from build123d import *

# Parameters (mm, degrees)
EXTRUDE_1_DEPTH     = 10
FILLET_1_R          = 20
SKETCH_2_R          = 18.75
CUT_EXTRUDE_1_DEPTH = 81.195074662
SKETCH_5_R          = 1.65
CUT_EXTRUDE_4_DEPTH = 81.195074662
SKETCH_6_R          = 1.65
CUT_EXTRUDE_5_DEPTH = 81.195074662
SKETCH_7_R          = 18.75
SKETCH_7_R_2        = 17.75
EXTRUDE_2_DEPTH     = 3
CUT_EXTRUDE_6_DEPTH = 10
FILLET_5_R          = 5
FILLET_6_R          = 3


with BuildPart() as part:
    # ｽｹｯﾁ1 → ﾎﾞｽ - 押し出し1 (new body)
    with BuildSketch(Plane.XY):
        with BuildLine():
            Line((57.5, -15), (57.5, 15))
            Line((57.5, 15), (48.35142739, 38.928092678))
            ThreePointArc((48.35142739, 38.928092678), (39.173878846, 50.59371648), (25, 55))
            Line((25, 55), (-25, 55))
            ThreePointArc((-25, 55), (-39.173878846, 50.59371648), (-48.35142739, 38.928092678))
            Line((-48.35142739, 38.928092678), (-57.5, 15))
            Line((-57.5, 15), (-57.5, -15))
            Line((-57.5, -15), (57.5, -15))
        make_face()
    extrude(amount=EXTRUDE_1_DEPTH)

    # ﾌｨﾚｯﾄ1
    fillet_1_edges = [part.edges().sort_by_distance(p)[0] for p in [
        (57.5, 15, 5),
        (-57.5, 15, 5),
    ]]
    fillet(fillet_1_edges, radius=FILLET_1_R)

    # ｽｹｯﾁ2 → ｶｯﾄ - 押し出し1 (cut, through all)
    with BuildSketch(Plane.XY.offset(10)):
        with Locations((25, 30)):
            Circle(SKETCH_2_R)
        with Locations(Location((-25, 30, 0), (0, 0, 180))):
            Circle(SKETCH_2_R)
    extrude(amount=-CUT_EXTRUDE_1_DEPTH, mode=Mode.SUBTRACT)

    # ｽｹｯﾁ5 → ｶｯﾄ - 押し出し4 (cut, through all)
    with BuildSketch(Plane(origin=(0, 0, 0), x_dir=(-1, 0, 0), z_dir=(0, 0, -1))):
        with Locations((-25, 51.75)):
            Circle(SKETCH_5_R)
        with Locations((-9.620427509, 45.379572491)):
            Circle(SKETCH_5_R)
        with Locations((-3.25, 30)):
            Circle(SKETCH_5_R)
        with Locations((-9.620427509, 14.620427509)):
            Circle(SKETCH_5_R)
        with Locations((-25, 8.25)):
            Circle(SKETCH_5_R)
        with Locations((-40.379572491, 14.620427509)):
            Circle(SKETCH_5_R)
        with Locations((-46.75, 30)):
            Circle(SKETCH_5_R)
        with Locations((-40.379572491, 45.379572491)):
            Circle(SKETCH_5_R)
        with Locations(Location((40.379572491, 45.379572491, 0), (0, 0, 180))):
            Circle(SKETCH_5_R)
        with Locations(Location((46.75, 30, 0), (0, 0, 180))):
            Circle(SKETCH_5_R)
        with Locations(Location((40.379572491, 14.620427509, 0), (0, 0, 180))):
            Circle(SKETCH_5_R)
        with Locations(Location((25, 8.25, 0), (0, 0, 180))):
            Circle(SKETCH_5_R)
        with Locations(Location((9.620427509, 14.620427509, 0), (0, 0, 180))):
            Circle(SKETCH_5_R)
        with Locations(Location((3.25, 30, 0), (0, 0, 180))):
            Circle(SKETCH_5_R)
        with Locations(Location((9.620427509, 45.379572491, 0), (0, 0, 180))):
            Circle(SKETCH_5_R)
        with Locations(Location((25, 51.75, 0), (0, 0, 180))):
            Circle(SKETCH_5_R)
    extrude(amount=-CUT_EXTRUDE_4_DEPTH, mode=Mode.SUBTRACT)

    # ｽｹｯﾁ6 → ｶｯﾄ - 押し出し5 (cut, through all)
    with BuildSketch(Plane(origin=(0, 0, 0), x_dir=(-1, 0, 0), z_dir=(0, 0, -1))):
        with Locations((-52.5, -5)):
            Circle(SKETCH_6_R)
        with Locations(Location((52.5, -5, 0), (0, 0, 180))):
            Circle(SKETCH_6_R)
        with Locations((0, -5)):
            Circle(SKETCH_6_R)
    extrude(amount=-CUT_EXTRUDE_5_DEPTH, mode=Mode.SUBTRACT)

    # ｽｹｯﾁ7 → ﾎﾞｽ - 押し出し2 (add)
    # profile 1 of 2: a face of its own
    with BuildSketch(Plane.XY.offset(10)):
        with Locations((-25, 30)):
            Circle(SKETCH_7_R)
        with Locations((-25, 30)):
            Circle(SKETCH_7_R_2, mode=Mode.SUBTRACT)
    # profile 2 of 2: a face of its own
    with BuildSketch(Plane.XY.offset(10)):
        with Locations((25, 30)):
            Circle(SKETCH_7_R)
        with Locations((25, 30)):
            Circle(SKETCH_7_R_2, mode=Mode.SUBTRACT)
    extrude(amount=-EXTRUDE_2_DEPTH)

    # ｽｹｯﾁ8 → ｶｯﾄ - 押し出し6 (cut)
    with BuildSketch(Plane(origin=(0, 0, 0), x_dir=(-1, 0, 0), z_dir=(0, 0, -1))):
        with BuildLine():
            Line((-42.5, -9), (-7.5, -9))
            Line((-7.5, -9), (-7.5, 8.786796564))
            ThreePointArc((-7.5, 8.786796564), (-25, 2.5), (-42.5, 8.786796564))
            Line((-42.5, 8.786796564), (-42.5, -9))
        make_face()
        with BuildLine():
            Line((42.5, -9), (42.5, 8.786796564))
            ThreePointArc((42.5, 8.786796564), (25, 2.5), (7.5, 8.786796564))
            Line((7.5, 8.786796564), (7.5, -9))
            Line((7.5, -9), (42.5, -9))
        make_face()
    extrude(amount=-CUT_EXTRUDE_6_DEPTH, mode=Mode.SUBTRACT)

    # ﾌｨﾚｯﾄ5
    fillet_5_edges = [part.edges().sort_by_distance(p)[0] for p in [
        (57.5, -15, 5),
        (-57.5, -15, 5),
    ]]
    fillet(fillet_5_edges, radius=FILLET_5_R)

    # ﾌｨﾚｯﾄ6
    fillet_6_edges = [part.edges().sort_by_distance(p)[0] for p in [
        (7.5, -9, 5),
        (7.5, 8.786796564, 5),
        (42.5, 8.786796564, 5),
        (42.5, -9, 5),
        (-42.5, 8.786796564, 5),
        (-7.5, 8.786796564, 5),
        (-7.5, -9, 5),
        (-42.5, -9, 5),
    ]]
    fillet(fillet_6_edges, radius=FILLET_6_R)


solid = part.part
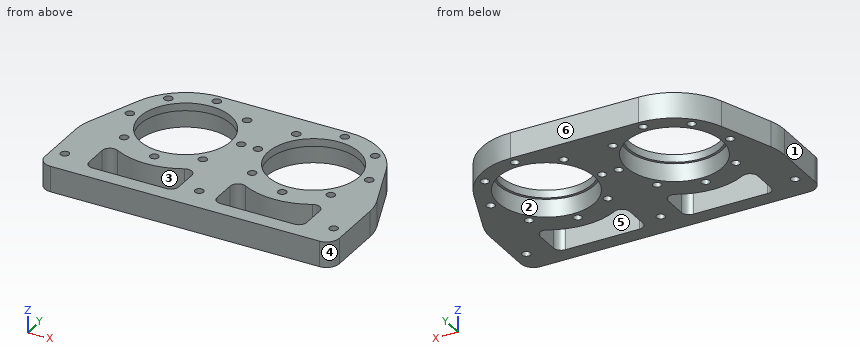
CAD build for the part. Positions are in the model's coordinates, mm. Face numbers are marked on the shaded views. A direction names the side the tool comes from. Give positions to 0.01 mm unless a question says otherwise; leave off trailing zeros. Write each loop counter-clockwise with the first axis right and the second up, starting at its lowest first coordinate (ties: lowest second). Pieces come first, ordered by that corner, then holes. Notation, with made-up numbers: M 27.25,87 L 74.25,87 A19 ccw 74.25,92 Z; hole C -7,30 d9. An arc over 180 degrees is marked long. Put each result on its own line as item: value. Start each with the question number.
(1) Band-saw the part on A-A, the plane x = 3.25. Write the cut outline in (y, z).
(2) Mould opens along Y. For the marked faces 4, 5 and 6 say: +Y half, -Y half, draft (parallel to the pull), parting line (faces both ways), or undercut.
(3) Flat gauge pins, fed straight in: pin 1 Ø1.5 at (x, z) = (-31.5, 1.5) entering from +Y; pin 2 Ø1.5 at (x, z) = (-30.5, 4.5) entering from +Y. Where does each tip first touch, or does it go through?
(4) Which spindle directions (+Z, -Z, +X, -X, +Y, -Y) get a long thin tool onto all of the face, cutting with end or side? Do the marked faces 1, 2 and 3. Say none if no direction does.
(5) Probe L1, parallel to Y at x = -25, z = 6.5; L2, parallel to X at y = -2, z = 9; L3, parallel to X at y = 9, z = 8.5. List the from-to ranges inside material, lowest first.
(6) Band-saw the part on B-B, the plane x = -28.5. Write the cut outline in (y, z).
(7) Band-saw the part on C-C, the plane x = 29.5. Write the cut outline in (y, z).
(8) Band-saw the part on D-D, the plane z = 4.75. Give the number of separate pieces and of enclosed holes in the cut face, and give its area (3 significant figures).
Response values:
1. outline: M -15,0 L 28.35,0 L 28.35,10 L -15,10 Z; M 31.65,0 L 55,0 L 55,10 L 31.65,10 Z
2. face 4: -Y half
2. face 5: undercut
2. face 6: +Y half
3. pin 1: stops at y = 54.33
3. pin 2: stops at y = 54.54
4. face 1: +Z, -Z, -X, +Y, -Y
4. face 2: -Z
4. face 3: +Z, -Z
5. L1: y = -15 to -9, 2.5 to 6.6, 9.9 to 11.25, 48.75 to 50.1, 53.4 to 55
5. L2: x = -57.5 to -42.5, -7.5 to 7.5, 42.5 to 57.5
5. L3: x = -57.5 to -26.47, -23.53 to 23.53, 26.47 to 57.5
6. outline: M -15,0 L -9,0 L -9,10 L -15,10 Z; M 2.72,0 L 11.58,0 L 11.58,7 L 12.6,7 L 12.6,10 L 2.72,10 Z; M 47.4,7 L 48.42,7 L 48.42,0 L 54.75,0 L 54.75,10 L 47.4,10 Z
7. outline: M -15,0 L -9,0 L -9,10 L -15,10 Z; M 2.87,0 L 11.8,0 L 11.8,7 L 12.83,7 L 12.83,10 L 2.87,10 Z; M 47.17,7 L 48.2,7 L 48.2,0 L 54.59,0 L 54.59,10 L 47.17,10 Z
8. separate pieces: 1
8. enclosed holes: 23
8. area: 4,040 mm2
